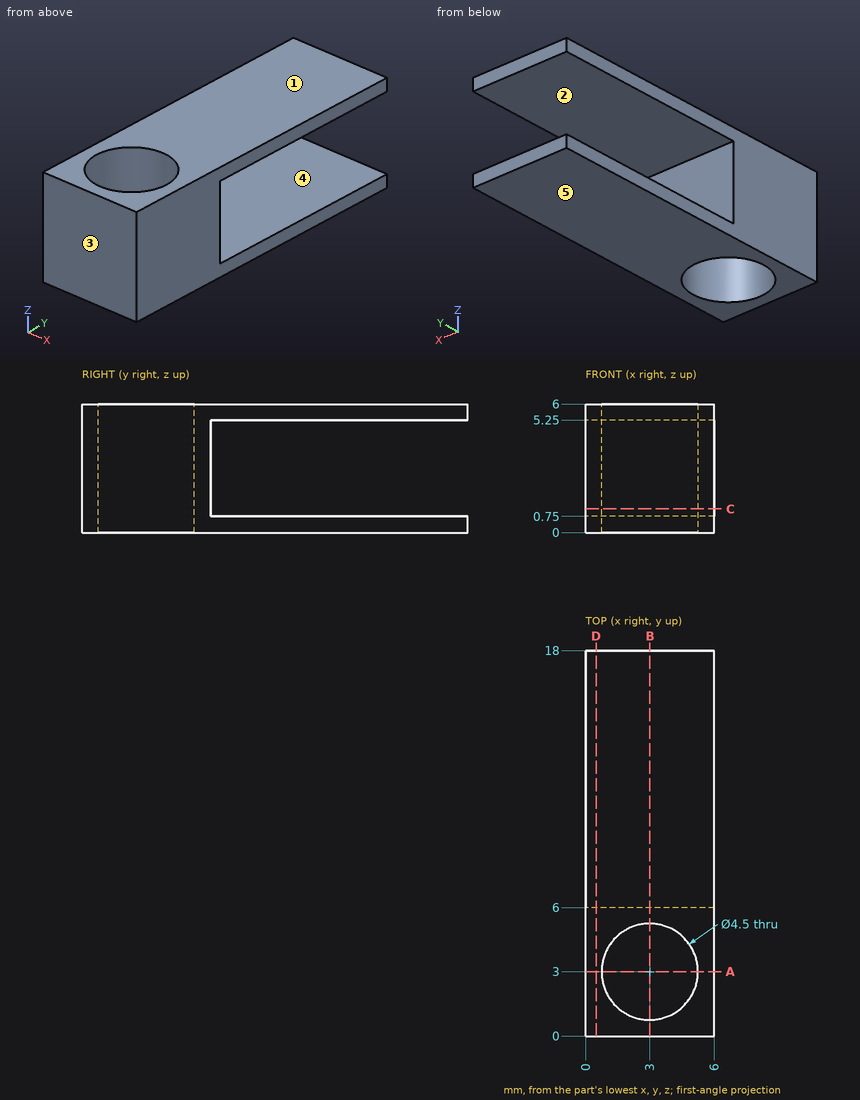
Design review of the part shown in the three views and the two pictorial views. Dimensions are in mm from the part's minimum x, y and z. A direction names the side the tool comes from. Round coordinates to 2 decimals unless told otherwise and drop trailing zeros. Loops run counter-clockwise (first coordinate to the right, second up) from the corner with the lowest first, then second, coordinate; pieces in that order, holes last. Notation, with made-up numbers: (-12.75, 87) -> (29.25, 87) arc R9 ccw to (29.25, 104) -> close; hole circle Ø8 at (16.5, 66.25). An arc over 180 degrees is marked (long way). Answer as a JSON object with one key per item and string values. Group by question number.
1) We need section D-D on x = 0.5. Write out the cut boundary in (y, z).
2) We need section C-C on z = 1.1. Write out the cut boundary in (x, y), then the cut area to 3 significant figures.
3) For the marked faces 1 and 2, list the 3-axis set-ups (+Z, -Z, +X, -X, +Y, -Y) from which the entire face can be reached by the end or side of a thin tool; tool diameter is ignored.
4) For pin 1 Ø1.5 at (x, z) = (2.5, 2.5) entering from +Y; pin 2 Ø1 at (y, z) = (14, 3) entering from +X, all flat-tipped, find the tip position at first contact; note any pin that passes through.
5) We need section A-A on y = 3. Write out the cut boundary in (x, z), then the cut area to 3 significant figures.
6) We need section B-B on x = 3. Write out the cut boundary in (y, z).
7) Mouldability with a two-part tool opening along Z and no side actions: class the marked faces 3, 4 and 5 as released by +Z, released by -Z, zero draft, split by the parting line, or undercut.
8) For line 1 (Z direction, x = 2.5, y = 10.5); line 2 (Y direction, x = 4.7, z = 3.7), list the stretches that pass through material, from the lowest coordinate up. Write a range as [from, to].
Result set:
{
 "1": {"outline": "(0, 0) -> (18, 0) -> (18, 0.75) -> (6, 0.75) -> (6, 5.25) -> (18, 5.25) -> (18, 6) -> (0, 6) -> close"},
 "2": {"outline": "(0, 0) -> (6, 0) -> (6, 6) -> (0, 6) -> close; hole circle Ø4.5 at (3, 3)", "area": "20.1 mm²"},
 "3": {"face 1": "+Z, +X, -X, +Y, -Y", "face 2": "+X, -X, +Y"},
 "4": {"pin 1": "y = 6", "pin 2": "through"},
 "5": {"outline": "(0, 0) -> (0.75, 0) -> (0.75, 6) -> (0, 6) -> close; (5.25, 0) -> (6, 0) -> (6, 6) -> (5.25, 6) -> close", "area": "9.00 mm²"},
 "6": {"outline": "(0, 0) -> (0.75, 0) -> (0.75, 6) -> (0, 6) -> close; (5.25, 0) -> (18, 0) -> (18, 0.75) -> (6, 0.75) -> (6, 5.25) -> (18, 5.25) -> (18, 6) -> (5.25, 6) -> close"},
 "7": {"face 3": "zero draft", "face 4": "undercut", "face 5": "released by -Z"},
 "8": {"line 1": "[0, 0.75], [5.25, 6]", "line 2": "[0, 1.53], [4.47, 6]"}
}
